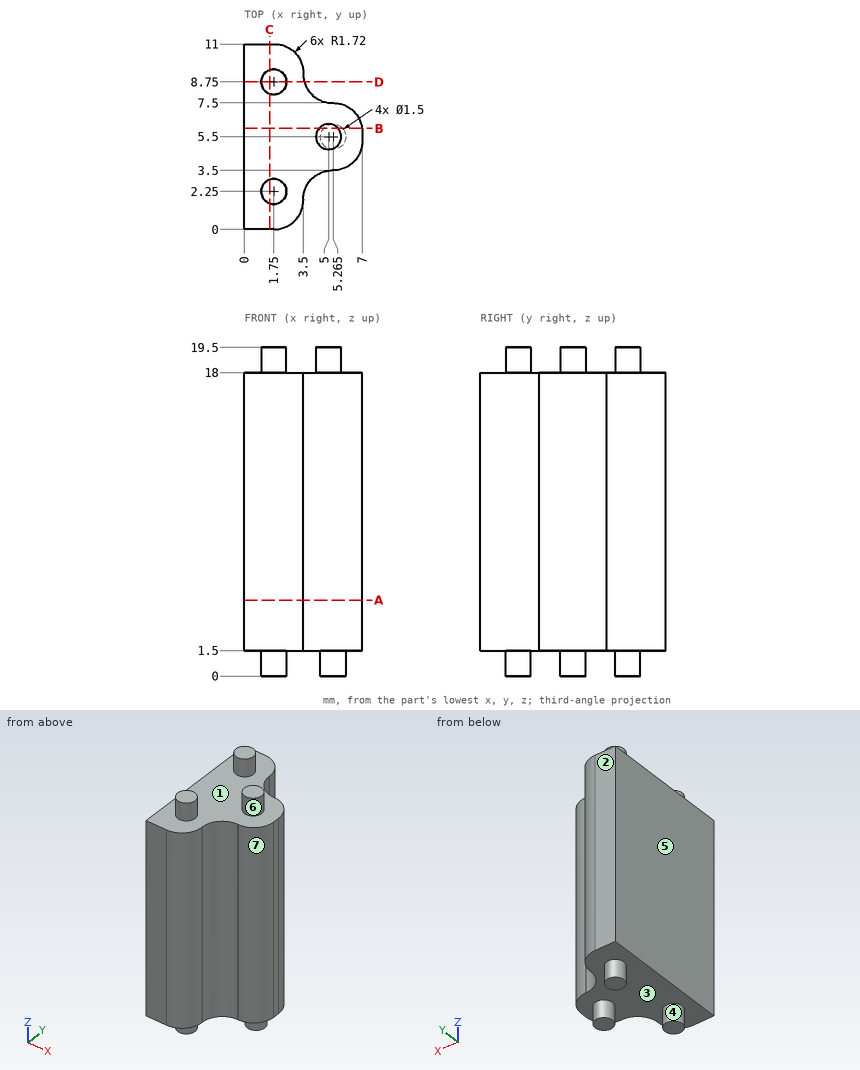
Geometry check sheet. Reference: drawing and pictorial views, mm from the part's lowest x, y, z. A direction names the side the tool comes from. Give positions to 0.01 mm unless a question says otherwise; leave off trailing zeros. Loops run counter-clockwise (first coordinate to the right, second up) from the corner with the lowest first, then second, coordinate; pieces in that order, holes last. Notation, with made-up numbers: (27, -38) - (75, -38) arc R9 cw to (75, -23) - close; hole circle Ø4 at (56, 73.25). An arc over 180 degrees is marked (long way). One line per question, with ' | ' between items. Start each with the question number.
1. Cross-section at C-C, the plane x = 1.5. Enter the section's corners in (y, z), plus the area to 3 significant figures.
2. Material ranges on line 1 along Z through (x, y) = (2.5, 1.5); line 2 along Y through (x, z) = (2.75, 5.25); line 3 along X through (y, z) = (8.5, 8), recorded low to high. Write a range as [from, to].
3. Set-up check for the marked faces 1, 2 and 3: record each of +Z, -Z, +X, -X, +Y, -Y from which the full face is reachable in a straight line by a thin tool's end or side.
4. Cross-section at D-D, the plane y = 8.75. Enter the section's corners in (x, z).
5. Cross-section at B-B, the plane y = 6. Enter the section's corners in (x, z), plus the area to 3 significant figures.
6. Cross-section at A-A, the plane z = 4.5. Enter the section's corners in (x, y).
7. Gauge pin test, flat ends, axial feed: pin 1 Ø2 at (x, y) = (4.5, 8.5) entering from -Z; pin 2 Ø3.5 at (x, y) = (2, 6) entering from +Z; pin 3 Ø2 at (x, z) = (3.5, 8.5) entering from +Y. Record the tip position at first contact, or that the pin passes through.
8. Draft check along Y on the marked faces 4, 5, 6 and 7. Enter one of: released by +Y, released by -Y, zero draft, split by the parting line, or undercut.
Check result:
1) outline: (0, 1.5) - (1.54, 1.5) - (1.54, 0) - (2.96, 0) - (2.96, 1.5) - (8.04, 1.5) - (8.04, 0) - (9.46, 0) - (9.46, 1.5) - (11, 1.5) - (11, 18) - (9.46, 18) - (9.46, 19.5) - (8.04, 19.5) - (8.04, 18) - (2.96, 18) - (2.96, 19.5) - (1.54, 19.5) - (1.54, 18) - (0, 18) - close | area: 190 mm2
2) line 1: z = [1.5, 18] | line 2: y = [0.3, 10.7] | line 3: x = [0, 3.66]
3) face 1: +Z | face 2: +Z, -Z, +X, -X, +Y | face 3: -Z
4) outline: (0, 1.5) - (1, 1.5) - (1, 0) - (2.5, 0) - (2.5, 1.5) - (3.57, 1.5) - (3.57, 18) - (2.5, 18) - (2.5, 19.5) - (1, 19.5) - (1, 18) - (0, 18) - close
5) outline: (0, 1.5) - (4.71, 1.5) - (4.71, 0) - (5.82, 0) - (5.82, 1.5) - (6.99, 1.5) - (6.99, 18) - (5.56, 18) - (5.56, 19.5) - (4.44, 19.5) - (4.44, 18) - (0, 18) - close | area: 119 mm2
6) outline: (0, 0) - (1.78, 0) arc R1.72 ccw to (3.5, 1.72) - (3.5, 1.78) arc R1.72 cw to (5.22, 3.5) - (5.28, 3.5) arc R1.72 ccw to (7, 5.22) - (7, 5.78) arc R1.72 ccw to (5.28, 7.5) - (5.22, 7.5) arc R1.72 cw to (3.5, 9.22) - (3.5, 9.28) arc R1.72 ccw to (1.78, 11) - (0, 11) - close
7) pin 1: stops at z = 1.5 | pin 2: stops at z = 18 | pin 3: stops at y = 10.84
8) face 4: undercut | face 5: zero draft | face 6: split by the parting line | face 7: released by -Y
